```python
from build123d import *

# Parameters (mm, degrees)
SKETCH1_R           = 3.911052803
BOSS_EXTRUDE1_DEPTH = 4
CAVITY1_START       = 0.003221124
CAVITY1_DEPTH       = 7.362862002


# Read off the part's stored shape, not the designer's step: Cavity1
with BuildPart() as part:
    # Sketch1 → Boss-Extrude1 (new body)
    with BuildSketch(Plane(origin=(0, 0, 0), x_dir=(1, 0, 0), z_dir=(0, 1, 0))):
        with BuildLine():
            Line((0, 0), (30, 0))
            Line((30, 0), (25.709430043, 75.411524479))
            ThreePointArc((25.709430043, 75.411524479), (22.592877256, 82.112613927), (15.725576294, 84.84348898))
            Line((15.725576294, 84.84348898), (15.172794511, 84.84348898))
            Line((15.172794511, 84.84348898), (14.566572295, 84.84348898))
            ThreePointArc((14.566572295, 84.84348898), (7.713312448, 82.125853257), (4.584985356, 75.450054873))
            Line((4.584985356, 75.450054873), (0, 0))
        make_face()
        with Locations(Location((15.172794511, 74.362549593, 0), (0, 0, 270))):
            Circle(SKETCH1_R, mode=Mode.SUBTRACT)
    extrude(amount=BOSS_EXTRUDE1_DEPTH)

    # Cavity1 outline → Cavity1 (cut)
    with BuildSketch(Plane(origin=(0, 0, 0), x_dir=(0.9990997712006259, -0.037322908087554375, 0.02016550814496959), z_dir=(0.042422248724659405, 0.8790035901407052, -0.4749242479942401)).offset(CAVITY1_START)):
        with BuildLine():
            ThreePointArc((20.385742614, -1.901408695), (10.614392107, 4.37266206), (-0.069777809, -0.176158423))
            Line((-0.069777809, -0.176158423), (-2, -2.55511847))
            Line((-2, -2.55511847), (-2, -3))
            Line((-2, -3), (21.005093085, -3))
            Line((21.005093085, -3), (20.385742614, -1.901408695))
        make_face()
    extrude(amount=CAVITY1_DEPTH, mode=Mode.SUBTRACT)


solid = part.part
```
Source: CAD feature listing. Evaluate the final solid. Frame: model axes, mm. Coordinates: 2 decimals unless noted, no trailing zeros. Order: outer loops, then holes, each group sorted by start corner. A loop starts at its lowest first (then second) coordinate and runs counter-clockwise, first axis right, second up. Notation, with made-up numbers: M 32,-22.5 L 60,-22.5 A25 ccw 60,14.5 Z; hole C 33,0 d3. An arc over 180 degrees is marked long. Write each question's results on one line, items separated by ' | '. Start each with the question number.
1) Section query B-B (x = 26.5). Return the cut outline in (y, z).
2) Section query C-C (z = -18.5). Return the cut outline in (x, y), plus the area to 3 significant figures.
3) Section query A-A (z = -72.5). Return the cut outline in (x, y).
4) Contact query for flat-ended pins moving along their axis: pin 1 Ø1 at (y, z) = (2, -26.5) entering from -X; pin 2 Ø2 at (x, y) = (10, 1.5) entering from -Z; pin 3 Ø6.5 at (x, z) = (15.17, -74.36) entering from +Y; pin 4 Ø2 at (y, z) = (2, -26.5) entering from +X. Output: stop coordinate, or through.
5) Line query: line 1 (Z direction, x = 16, y = 3.3); line 2 (Z direction, x = 12.5, y = 0.35); line 3 (X direction, y = 1.8, z = -3.5). Output: solid intervals per line, ascending. Write a range as from..to.
6) Draft query along X for faces 1 (the face through (22.67, 1.97, -82.04)), 2 (the face through (15.34, 1.97, -78.27)), 3 (the face through (24, 2, 0)). Return one class per face: released by +X, released by -X, zero draft, split by the parting line, or undercut.
Answers:
1) outline: M 0,-61.52 L 4,-61.52 L 4,0 L 0,0 Z
2) outline: M 1.12,0 L 28.95,0 L 28.95,4 L 1.12,4 Z | area: 111 mm^2
3) outline: M 4.41,0 L 11.73,0 L 11.73,4 L 4.41,4 Z; M 18.61,0 L 25.88,0 L 25.88,4 L 18.61,4 Z
4) pin 1: stops at x = 1.58 | pin 2: stops at z = -84.19 | pin 3: passes through | pin 4: stops at x = 28.55
5) line 1: z = -84.84..-78.19, -70.54..-4.92 | line 2: z = -84.63..-77.22, -71.51..-4.84 | line 3: x = 0.21..2.67, 16.77..29.8
6) face 1: released by +X | face 2: undercut | face 3: zero draft
